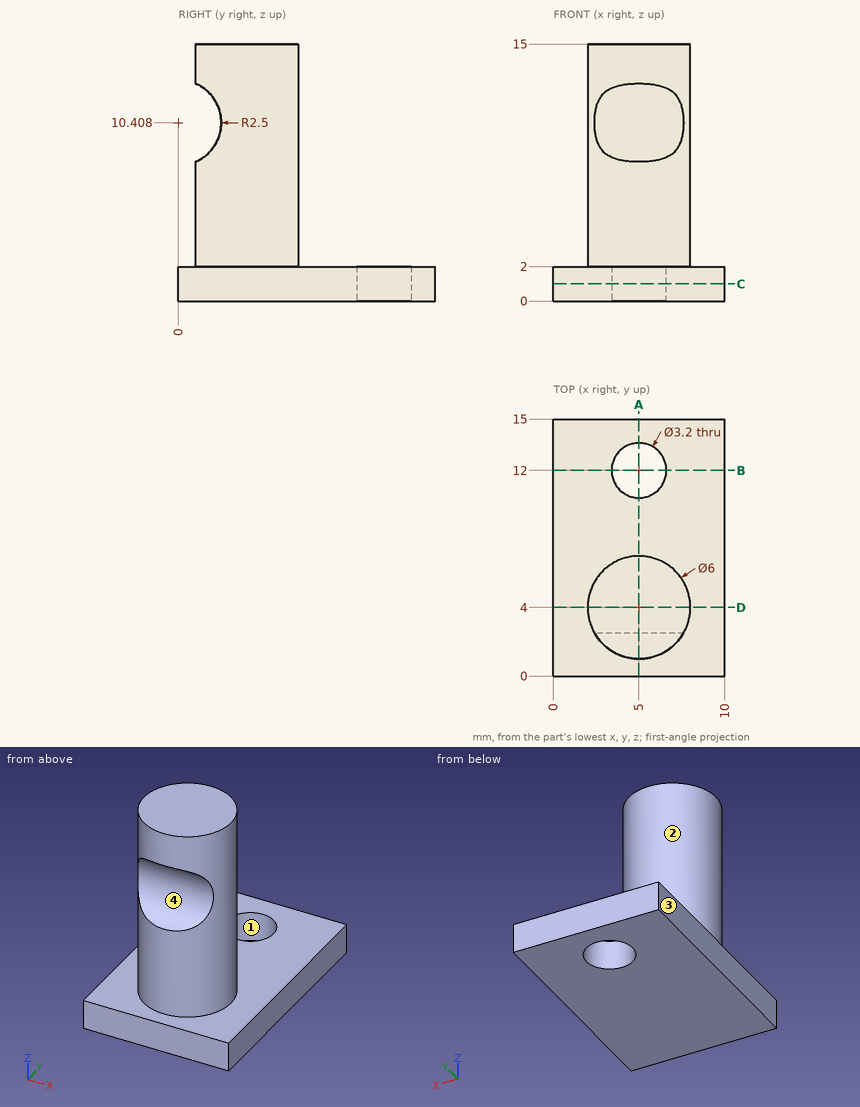
Can you work these out from the drawing? Everything is in mm from the part's minimum corner. Round coordinates to 2 decimals unless told otherwise and drop trailing zeros. Loops run counter-clockwise (first coordinate to the right, second up) from the corner with the lowest first, then second, coordinate; pieces in that order, holes last. Notation, with made-up numbers: M -33.75,3.25 L -29.75,3.25 A21 cw -29.75,42.25 Z; hole C 57,86 d7. An arc over 180 degrees is marked long. Answer in a Markdown table with one row per item.
1. I'm going to push flat-ended pins straight in: pin 1 Ø3 at (x, y) = (5, 12) entering from +Z; pin 2 Ø5 at (x, z) = (5, 7) entering from -Y. Where does each tip first touch, or does it pass through?
Established:
| item | result |
|---|---|
| pin 1 | through |
| pin 2 | y = 1 |
2. Please list where these lines run through material, in increasing order: line 1 (Y direction, x = 5, z = 1); line 2 (Z direction, x = 3.75, y = 14); line 3 (Y direction, x = 6, z = 0.5). Write a range as from..to.
Established:
| item | result |
|---|---|
| line 1 | 0..10.4, 13.6..15 |
| line 2 | 0..2 |
| line 3 | 0..10.75, 13.25..15 |
3. Thinking about a two-plate mould opening in X: for the marked faces 1, 2, 3 and 4, which applies, pulls with the +X half, pulls with the -X half, needs draft (parallel to the pull), parting line crosses it, or undercut?
Established:
| item | result |
|---|---|
| face 1 | undercut |
| face 2 | parting line crosses it |
| face 3 | pulls with the -X half |
| face 4 | needs draft |
4. If we section it at C-C, the plane z = 1: Please give me the cut outline in (x, y), plus the area to 3 significant figures.
Established:
| item | result |
|---|---|
| outline | M 0,0 L 10,0 L 10,15 L 0,15 Z; hole C 5,12 d3.2 |
| area | 142 mm² |
5. If we section it at D-D, the plane y = 4: Please give me the cut outline in (x, z), plus the area to 3 significant figures.
Established:
| item | result |
|---|---|
| outline | M 0,0 L 10,0 L 10,2 L 8,2 L 8,15 L 2,15 L 2,2 L 0,2 Z |
| area | 98.0 mm² |
6. If we section it at A-A, the plane x = 5: Please give me the cut outline in (y, z).
Established:
| item | result |
|---|---|
| outline | M 0,0 L 10.4,0 L 10.4,2 L 7,2 L 7,15 L 1,15 L 1,12.7 A2.5 cw 1,8.12 L 1,2 L 0,2 Z; M 13.6,0 L 15,0 L 15,2 L 13.6,2 Z |
7. If we section it at B-B, the plane y = 12: Please give me the cut outline in (x, z).
Established:
| item | result |
|---|---|
| outline | M 0,0 L 3.4,0 L 3.4,2 L 0,2 Z; M 6.6,0 L 10,0 L 10,2 L 6.6,2 Z |
